Verification items for the finished model (mm, model axes). A direction names the side the tool comes from. Give positions to 0.01 mm unless a question says otherwise; leave off trailing zeros. Write each loop counter-clockwise with the first axis right and the second up, starting at its lowest first coordinate (ties: lowest second). Pieces come first, ordered by that corner, then holes. Notation, with made-up numbers: (-26, 50.5) -> (33, 50.5) arc R27 ccw to (33, 89.5) -> close; hole circle Ø10 at (59.25, 68.5). An arc over 180 degrees is marked (long way). Write item = value, one per line.
from build123d import *

# Parameters (mm, degrees)
SKETCH_1_R          = 1.5
SKETCH_1_W          = 41
SKETCH_1_H          = 20
EXTRUDE_1_DEPTH     = 5
SKETCH_6_R          = 6
SKETCH_6_R_2        = 4
EXTRUDE_3_DEPTH     = 15
SKETCH_7_R          = 2.5
CUT_EXTRUDE_1_DEPTH = 76.573459736


with BuildPart() as part:
    # 草图1 → 凸台-拉伸1 (new body)
    with BuildSketch(Plane.XY):
        with BuildLine():
            Line((50.475318096, 32.112170347), (50.475318096, -29.083982076))
            ThreePointArc((50.475318096, -29.083982076), (49.59663844, -31.205302419), (47.475318096, -32.083982076))
            Line((47.475318096, -32.083982076), (-46.199426394, -32.083982076))
            ThreePointArc((-46.199426394, -32.083982076), (-48.320746738, -31.205302419), (-49.199426394, -29.083982076))
            Line((-49.199426394, -29.083982076), (-49.199426394, -17.478939569))
            ThreePointArc((-49.199426394, -17.478939569), (-49.22509181, -17.087360992), (-49.301648916, -16.702482433))
            Line((-49.301648916, -16.702482433), (-61.198360071, 27.696648043))
            ThreePointArc((-61.198360071, 27.696648043), (-60.680642613, 30.299389465), (-58.300582592, 31.473105178))
            Line((-58.300582592, 31.473105178), (-2.524681904, 31.473105178))
            ThreePointArc((-2.524681904, 31.473105178), (-0.40336156, 32.351784835), (0.475318096, 34.473105178))
            Line((0.475318096, 34.473105178), (0.475318096, 38.576271962))
            ThreePointArc((0.475318096, 38.576271962), (1.353997752, 40.697592306), (3.475318096, 41.576271962))
            Line((3.475318096, 41.576271962), (43.743267288, 41.576271962))
            ThreePointArc((43.743267288, 41.576271962), (45.243267288, 41.174348173), (46.3413435, 40.076271962))
            Line((46.3413435, 40.076271962), (50.073394307, 33.612170347))
            ThreePointArc((50.073394307, 33.612170347), (50.373095575, 32.888627482), (50.475318096, 32.112170347))
        make_face()
        with Locations((34.275318096, -0.183982076)):
            Circle(SKETCH_1_R, mode=Mode.SUBTRACT)
        with Locations((34.275318096, -9.983982076)):
            Circle(SKETCH_1_R, mode=Mode.SUBTRACT)
        with Locations(Location((-14.324681904, -9.983982076, 0), (0, 0, 180))):
            Circle(SKETCH_1_R, mode=Mode.SUBTRACT)
        with Locations(Location((-14.324681904, -0.183982076, 0), (0, 0, 180))):
            Circle(SKETCH_1_R, mode=Mode.SUBTRACT)
        with Locations((45.475318096, -26.083982076)):
            Circle(SKETCH_1_R, mode=Mode.SUBTRACT)
        with Locations((45.475318096, 28.916017924)):
            Circle(SKETCH_1_R, mode=Mode.SUBTRACT)
        with Locations((-44.524681904, -26.083982076)):
            Circle(SKETCH_1_R, mode=Mode.SUBTRACT)
        with Locations((-54.524681904, 28.916017924)):
            Circle(SKETCH_1_R, mode=Mode.SUBTRACT)
        with Locations((34.275318096, 10.916017924)):
            Circle(SKETCH_1_R, mode=Mode.SUBTRACT)
        with Locations((-22.724681904, 10.916017924)):
            Circle(SKETCH_1_R, mode=Mode.SUBTRACT)
        with Locations((34.275318096, -19.083982076)):
            Circle(SKETCH_1_R, mode=Mode.SUBTRACT)
        with Locations((-22.724681904, -19.083982076)):
            Circle(SKETCH_1_R, mode=Mode.SUBTRACT)
        with Locations((9.975318096, -5.083982076)):
            Rectangle(SKETCH_1_W, SKETCH_1_H, mode=Mode.SUBTRACT)
        with BuildLine():
            Line((43.743267288, 24.388896624), (43.743267288, 13.793120092))
            ThreePointArc((43.743267288, 13.793120092), (41.751826733, 10.967733774), (38.421395391, 11.893406721))
            Line((38.421395391, 11.893406721), (29.752123683, 22.489183253))
            ThreePointArc((29.752123683, 22.489183253), (29.362986533, 25.673587226), (32.07399558, 27.388896624))
            Line((32.07399558, 27.388896624), (40.743267288, 27.388896624))
            ThreePointArc((40.743267288, 27.388896624), (42.864587632, 26.510216968), (43.743267288, 24.388896624))
        make_face(mode=Mode.SUBTRACT)
        with BuildLine():
            Line((27.205627867, 8.388896624), (18.282890218, 8.388896624))
            ThreePointArc((18.282890218, 8.388896624), (16.161569875, 9.26757628), (15.282890218, 11.388896624))
            Line((15.282890218, 11.388896624), (15.282890218, 22.294464861))
            ThreePointArc((15.282890218, 22.294464861), (17.274330774, 25.11985118), (20.604762116, 24.194178232))
            Line((20.604762116, 24.194178232), (29.527499765, 13.288609995))
            ThreePointArc((29.527499765, 13.288609995), (29.916636915, 10.104206022), (27.205627867, 8.388896624))
        make_face(mode=Mode.SUBTRACT)
        with BuildLine():
            Line((-2.92600442, 27.388896624), (5.743267288, 27.388896624))
            ThreePointArc((5.743267288, 27.388896624), (7.864587632, 26.510216968), (8.743267288, 24.388896624))
            Line((8.743267288, 24.388896624), (8.743267288, 13.793120092))
            ThreePointArc((8.743267288, 13.793120092), (6.751826733, 10.967733774), (3.421395391, 11.893406721))
            Line((3.421395391, 11.893406721), (-5.247876317, 22.489183253))
            ThreePointArc((-5.247876317, 22.489183253), (-5.637013467, 25.673587226), (-2.92600442, 27.388896624))
        make_face(mode=Mode.SUBTRACT)
        with BuildLine():
            Line((-7.794372133, 8.388896624), (-16.717109782, 8.388896624))
            ThreePointArc((-16.717109782, 8.388896624), (-18.838430125, 9.26757628), (-19.717109782, 11.388896624))
            Line((-19.717109782, 11.388896624), (-19.717109782, 22.294464861))
            ThreePointArc((-19.717109782, 22.294464861), (-17.725669226, 25.11985118), (-14.395237884, 24.194178232))
            Line((-14.395237884, 24.194178232), (-5.472500235, 13.288609995))
            ThreePointArc((-5.472500235, 13.288609995), (-5.083363085, 10.104206022), (-7.794372133, 8.388896624))
        make_face(mode=Mode.SUBTRACT)
        with BuildLine():
            Line((-38.13984743, 8.388896624), (-29.217109782, 8.388896624))
            ThreePointArc((-29.217109782, 8.388896624), (-27.095789438, 9.26757628), (-26.217109782, 11.388896624))
            Line((-26.217109782, 11.388896624), (-26.217109782, 22.294464861))
            ThreePointArc((-26.217109782, 22.294464861), (-28.208550337, 25.11985118), (-31.538981679, 24.194178232))
            Line((-31.538981679, 24.194178232), (-40.461719328, 13.288609995))
            ThreePointArc((-40.461719328, 13.288609995), (-40.850856478, 10.104206022), (-38.13984743, 8.388896624))
        make_face(mode=Mode.SUBTRACT)
        with BuildLine():
            Line((43.656664748, 38.726271962), (44.234015017, 37.726271962))
            ThreePointArc((44.234015017, 37.726271962), (44.234015017, 37.226271962), (43.801002315, 36.976271962))
            Line((43.801002315, 36.976271962), (4.377241885, 36.976271962))
            ThreePointArc((4.377241885, 36.976271962), (4.023688494, 37.122718571), (3.877241885, 37.476271962))
            Line((3.877241885, 37.476271962), (3.877241885, 38.476271962))
            ThreePointArc((3.877241885, 38.476271962), (4.023688494, 38.829825353), (4.377241885, 38.976271962))
            Line((4.377241885, 38.976271962), (43.223652046, 38.976271962))
            ThreePointArc((43.223652046, 38.976271962), (43.473652046, 38.909284664), (43.656664748, 38.726271962))
        make_face(mode=Mode.SUBTRACT)
        with BuildLine():
            Line((45.567840808, 34.916017924), (4.377241885, 34.916017924))
            ThreePointArc((4.377241885, 34.916017924), (4.023688494, 34.769571315), (3.877241885, 34.416017924))
            Line((3.877241885, 34.416017924), (3.877241885, 33.416017924))
            ThreePointArc((3.877241885, 33.416017924), (4.023688494, 33.062464534), (4.377241885, 32.916017924))
            Line((4.377241885, 32.916017924), (46.145191077, 32.916017924))
            ThreePointArc((46.145191077, 32.916017924), (46.578203779, 33.166017924), (46.578203779, 33.666017924))
            Line((46.578203779, 33.666017924), (46.00085351, 34.666017924))
            ThreePointArc((46.00085351, 34.666017924), (45.817840808, 34.849030626), (45.567840808, 34.916017924))
        make_face(mode=Mode.SUBTRACT)
    extrude(amount=EXTRUDE_1_DEPTH)

    # 草图6 → 凸台-拉伸3 (add)
    with BuildSketch(Plane.XY.offset(5)):
        with Locations(Location((-40.836658363, 23.267301815, 0), (0, 0, 180))):
            Circle(SKETCH_6_R)
        with Locations((-40.836658363, 23.267301815)):
            Circle(SKETCH_6_R_2, mode=Mode.SUBTRACT)
    extrude(amount=EXTRUDE_3_DEPTH)

    # 草图7 → 切除-拉伸1 (cut, through all)
    with BuildSketch(Plane.XY.offset(5)):
        with Locations((-40.836658363, 23.267301815)):
            Circle(SKETCH_7_R)
    extrude(amount=-CUT_EXTRUDE_1_DEPTH, mode=Mode.SUBTRACT)


solid = part.part
Item 1: Mould release check, pull along Y, two halves, no side actions. Record for faces 1 (the flat face through (48.18, 36.89, 2.46)), 2 (the flat face through (1, -32.084, 2)), 3 (the cylindrical face through (-17.774, 25.102, 2.465)): +Y half, -Y half, draft (parallel to the pull), parting line (faces both ways), or undercut.
Response values:
face_1 = +Y half
face_2 = -Y half
face_3 = undercut
Item 2: Set-up check for faces 4 (the flat face through (1, 27.389, 2)), 5 (the flat face through (-55.167, 5.186, 2.465)): record each of +Z, -Z, +X, -X, +Y, -Y from which the full face is reachable in a straight line by a thin tool's end or side.
Response values:
face_4 = +Z, -Z
face_5 = +Z, -Z, -X, -Y
Item 3: Sectioned sample at A-A on x = 26. Record the cut outline in (y, z), then the cut area to 3 significant figures.
Response values:
outline = (-32.08, 0) -> (-15.08, 0) -> (-15.08, 5) -> (-32.08, 5) -> close; (4.92, 0) -> (8.39, 0) -> (8.39, 5) -> (4.92, 5) -> close; (17.6, 0) -> (32.92, 0) -> (32.92, 5) -> (17.6, 5) -> close; (34.92, 0) -> (36.98, 0) -> (36.98, 5) -> (34.92, 5) -> close; (38.98, 0) -> (41.58, 0) -> (41.58, 5) -> (38.98, 5) -> close
area = 202 mm^2
Item 4: Go/stop test with flat-tipped pins: P1, Ø4, axis at x = 7, y = 13.5, coming from the +Z side; P2, Ø3, axis at y = 12, z = 4.5, coming from the -X side; P3, Ø8, axis at y = 19, z = 7, coming from the +X side; P4, Ø2.5, axis at y = 16.5, z = 2.5, coming from the -X side. Record where each tip stops, or that it passes through.
Response values:
P1 = 5
P2 = -57.39
P3 = 50.48
P4 = -58.53
Item 5: Sectioned sample at C-C on y = -22.5. Record the cut outline in (x, z), then the cut area to 3 significant figures.
Response values:
outline = (-49.2, 0) -> (50.48, 0) -> (50.48, 5) -> (-49.2, 5) -> close
area = 498 mm^2
Item 6: Material ranges on line 1 (Y direction, x = 15, z = 2.5); line 2 (X direction, y = 23, z = 14.75); line 3 (Y direction, x = 29, z = 4.5), recorded low to high.
Response values:
line_1 = -32.08 to -15.08, 4.92 to 32.92, 34.92 to 36.98, 38.98 to 41.58
line_2 = -46.83 to -44.83, -36.85 to -34.84
line_3 = -32.08 to -15.08, 4.92 to 8.98, 13.93 to 32.92, 34.92 to 36.98, 38.98 to 41.58
Item 7: Sectioned sample at D-D on z = 12.25. Record the cut outline in (x, y), then the cut area to 3 significant figures.
Response values:
outline = circle Ø12 at (-40.84, 23.27); hole circle Ø8 at (-40.84, 23.27)
area = 62.8 mm^2
Item 8: Sectioned sample at B-B on z = 1.5. Give the number of separate pieces and of enclosed holes in the cut face, then the cut area to 3 significant figures.
Response values:
separate_pieces = 1
enclosed_holes = 21
area = 5,150 mm^2
